from build123d import *

# Parameters (mm, degrees)
F1_DEPTH    = 4
F2_W        = 9.5
F2_H        = 8.5
F3_DEPTH    = 4
F4_R        = 1.75
F5_DEPTH    = 154
F6_R        = 10
F7_R        = 2
F8_R        = 2
F9_T1_DEPTH = 26.6944612474
F9_T3_DEPTH = 26.6917420766


# Not quite as in the source:
# - a fillet or chamfer that OpenCascade refuses, or shapes differently, is made with other operations: its cross-section is extruded or revolved along the edge and cut away or added
# - an extrude ends at something that could not be found from the text; its depth is read off the source's solid


with BuildPart() as f1:
    # F0 (on Top) → F1 (new body)
    with BuildSketch(Plane.XY):
        Polygon((-82.859264966, -11), (-85, -7.7888974491), (-88.3282011774, -10.007698234), (-85, -15), (-63.6905180954, -15), (-48.6905180954, -4), (-1.3094819046, -4), (13.6905180954, -15), (35, -15), (38.3282011774, -10.007698234), (35, -7.7888974491), (32.859264966, -11), (15, -11), (0, 0), (-50, 0), (-65, -11), align=None)
    extrude(amount=F1_DEPTH)

    # F2 (on face) → F3 (join, through all)
    with BuildSketch(Plane(origin=(0, 0, 0), x_dir=(-1, 0, 0), z_dir=(0, 1, 0))):
        with Locations((9.1, 4.25)):
            Rectangle(F2_W, F2_H)
        with Locations((40.9, 4.25)):
            Rectangle(F2_W, F2_H)
    extrude(amount=-F3_DEPTH)

    # F4 (on face) → F5 (cut, through all)
    with BuildSketch(Plane(origin=(0, 0, 0), x_dir=(-1, 0, 0), z_dir=(0, 1, 0))):
        with Locations((9.1, 3.75)):
            Circle(F4_R)
        with Locations((40.9, 3.75)):
            Circle(F4_R)
    extrude(amount=-F5_DEPTH, mode=Mode.SUBTRACT)

    # F6
    f6_edges = [f1.edges().sort_by_distance(p)[0] for p in [
        (35, -15, 2),
        (13.690518, -15, 2),
        (-63.690518, -15, 2),
        (-85, -15, 2),
        (-48.690518, -4, 2),
        (-1.309482, -4, 2),
    ]]
    fillet(f6_edges, radius=F6_R)

    # F7
    f7_edges = [f1.edges().sort_by_distance(p)[0] for p in [
        (35, -7.788897, 2),
        (-85, -7.788897, 2),
        (-65, -11, 2),
        (-82.859265, -11, 2),
        (32.859265, -11, 2),
        (15, -11, 2),
        (0, 0, 2),
        (-50, 0, 2),
    ]]
    fillet(f7_edges, radius=F7_R)

    # F8
    f8_edges = [f1.edges().sort_by_distance(p)[0] for p in [
        (-45.65, -2.00136, 4),
        (-13.85, -2, 4),
        (-4.35, -2.00136, 4),
        (-36.15, -2, 4),
    ]]
    fillet(f8_edges, radius=F8_R)

    # F9: fillet of radius 5 on 4 edges, made by hand

    # F9_s2 → F9_t1 (cut)
    with BuildSketch(Plane.XZ.offset(-11.3458710383)):
        with BuildLine():
            ThreePointArc((-41.1116515847, 8.5), (-43.9463851322, 7.6187723552), (-45.7819004528, 5.2857142857))
            Line((-45.7819004528, 5.2857142857), (-46.2489253396, 5.4642857143))
            ThreePointArc((-46.2489253396, 5.4642857143), (-46.15, 6), (-46.15, 8.5))
            Line((-46.15, 8.5), (-45.65, 9))
            Line((-45.65, 9), (-41.1116515847, 9))
            Line((-41.1116515847, 9), (-41.1116515847, 8.5))
        make_face()
        with BuildLine():
            ThreePointArc((-4.2180995472, 5.2857142857), (-6.0536148677, 7.6187723552), (-8.8883484153, 8.5))
            Line((-8.8883484153, 8.5), (-8.8883484153, 9))
            Line((-8.8883484153, 9), (-4.35, 9))
            Line((-4.35, 9), (-3.85, 8.5))
            ThreePointArc((-3.85, 8.5), (-3.85, 6), (-3.7510746604, 5.4642857143))
            Line((-3.7510746604, 5.4642857143), (-4.2180995472, 5.2857142857))
        make_face()
    extrude(amount=F9_T1_DEPTH, mode=Mode.SUBTRACT)

    # F9_s4 → F9_t3 (cut)
    with BuildSketch(Plane.XZ.offset(-11.3458710383)):
        with BuildLine():
            ThreePointArc((-36.0180995472, 5.2857142857), (-37.8536148677, 7.6187723552), (-40.6883484153, 8.5))
            Line((-40.6883484153, 8.5), (-40.6883484153, 9))
            Line((-40.6883484153, 9), (-36.15, 9))
            Line((-36.15, 9), (-35.65, 8.5))
            ThreePointArc((-35.65, 8.5), (-35.65, 6), (-35.5510746604, 5.4642857143))
            Line((-35.5510746604, 5.4642857143), (-36.0180995472, 5.2857142857))
        make_face()
        with BuildLine():
            ThreePointArc((-9.3116515847, 8.5), (-12.1463851322, 7.6187723552), (-13.9819004528, 5.2857142857))
            Line((-13.9819004528, 5.2857142857), (-14.4489253396, 5.4642857143))
            ThreePointArc((-14.4489253396, 5.4642857143), (-14.35, 6), (-14.35, 8.5))
            Line((-14.35, 8.5), (-13.85, 9))
            Line((-13.85, 9), (-9.3116515847, 9))
            Line((-9.3116515847, 9), (-9.3116515847, 8.5))
        make_face()
    extrude(amount=F9_T3_DEPTH, mode=Mode.SUBTRACT)


solid = f1.part
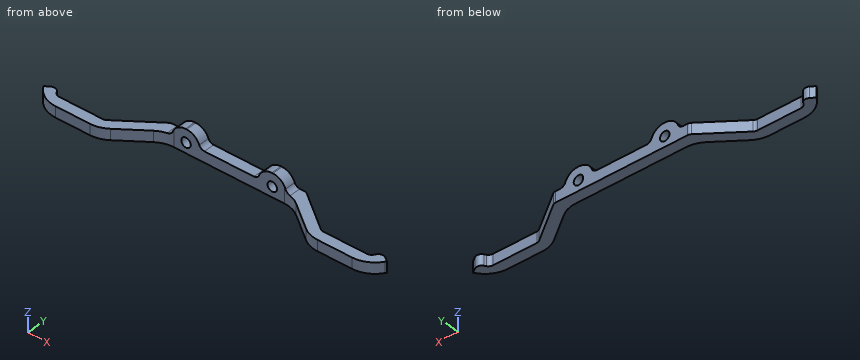
The listing builds one solid part. Answer for the finished solid, in the listing's coordinates (mm). Round coordinates to 2 decimals unless told otherwise and drop trailing zeros. Loops run counter-clockwise (first coordinate to the right, second up) from the corner with the lowest first, then second, coordinate; pieces in that order, holes last. Notation, with made-up numbers: M 35.5,1.5 L 91.5,1.5 A8 ccw 91.5,6.5 Z; hole C 78.5,57.5 d1. An arc over 180 degrees is marked long. Write each question's results on one line, items separated by ' | '. Start each with the question number.
1) Straight lines are drawn through the part: probe 1 along Z at (x, y) = (-9.1, -3.1); probe 2 along Y at (x, z) = (29.5, 3.5); probe 3 along X at (y, z) = (-6.5, 2.25). For each, find the intervals that lie inside material, in ascending order.
2) Find section B-B on x = -29.5. Write down the section's boundary in (y, z).
3) Find section C-C on x = 2.5. Write down the section's boundary in (y, z), plus the area to 3 significant figures.
4) Find section A-A on z = 7.25. Write down the section's boundary in (x, y), plus the area to 3 significant figures.
5) Each of these flat-tipped pins is pushed along its axis until it touches: pin 1 (4.5 mm diameter, centred on x = -9.1, z = 3.75, fed in from -Y); pin 2 (3 mm diameter, centred on y = -7.5, z = 6, fed in from +X); pin 3 (4.5 mm diameter, centred on x = -77, z = 1.5, fed in from +Y); pin 4 (4.5 mm diameter, centred on x = 12.5, y = -9.5, fed in from +Z). Where does it stop, or does it pass through?
Final values:
1) probe 1: 0 to 2, 5.5 to 8.5 | probe 2: -15 to -11 | probe 3: -58.86 to -52.1, 2.1 to 8.86
2) outline: M -4,0 L 0,0 L 0,4 L -4,4 Z
3) outline: M -6.79,0 L -1.83,0 L -1.83,4 L -6.79,4 Z | area: 19.8 mm²
4) outline: M -44.42,-4 L -37.38,-4 L -37.38,0 L -44.42,0 Z; M -12.62,-4 L -5.58,-4 L -5.58,0 L -12.62,0 Z | area: 56.3 mm²
5) pin 1: y = -4 | pin 2: through | pin 3: y = -11 | pin 4: z = 4
